```python
from build123d import *

# Parameters (mm, degrees)
MODEL_R             = 1.45
MODEL_RX            = 8.4
MODEL_RY            = 8
MODEL_W             = 3.6
MODEL_H             = 6.1
BOSS_EXTRUDE1_DEPTH = 5.85
FILLET1_R           = 0.3
FILLET2_R           = 1


with BuildPart() as part:
    # Model → Boss-Extrude1 (new body)
    with BuildSketch(Plane.XY):
        with BuildLine():
            Line((540.7427075, 594.649674665), (549.596103149, 594.649674665))
            Line((549.596103149, 594.649674665), (549.596103149, 592.109674665))
            Line((549.596103149, 592.109674665), (559.756103149, 592.109674665))
            Line((559.756103149, 592.109674665), (559.756103149, 594.649674665))
            Line((559.756103149, 594.649674665), (568.609498798, 594.649674665))
            ThreePointArc((568.609498798, 594.649674665), (575.419225536, 591.943953999), (578.10077955, 585.124674665))
            add(Edge.make_bspline(
                [(578.10077955, 585.124674665), (577.425296665, 565.444526899), (567.160030567, 565.124674665)],
                knots=[0, 0, 0, 1, 1, 1], degree=2))
            Line((567.160030567, 565.124674665), (542.192175731, 565.124674665))
            add(Edge.make_bspline(
                [(531.251426748, 585.124674665), (531.926909632, 565.444526899), (542.192175731, 565.124674665)],
                knots=[0, 0, 0, 1, 1, 1], degree=2))
            ThreePointArc((531.251426748, 585.124674665), (533.932980762, 591.943953999), (540.7427075, 594.649674665))
        make_face()
        with Locations((545.226103149, 571.324674665)):
            Circle(MODEL_R, mode=Mode.SUBTRACT)
        with Locations((564.126103149, 571.324674665)):
            Circle(MODEL_R, mode=Mode.SUBTRACT)
        with Locations(Location((541.476103149, 584.734674665), (0, 0, 180))):
            Ellipse(MODEL_RX, MODEL_RY, mode=Mode.SUBTRACT)
        with Locations(Location((567.876103149, 584.734674665), (0, 0, -180))):
            Ellipse(MODEL_RX, MODEL_RY, mode=Mode.SUBTRACT)
        with BuildLine():
            Line((549.856103149, 574.334674665), (554.676103149, 574.334674665))
            Line((554.676103149, 574.334674665), (559.496103149, 574.334674665))
            ThreePointArc((559.496103149, 574.334674665), (559.97693576, 574.533842054), (560.176103149, 575.014674665))
            Line((560.176103149, 575.014674665), (560.176103149, 578.654674665))
            ThreePointArc((560.176103149, 578.654674665), (559.97693576, 579.135507276), (559.496103149, 579.334674665))
            Line((559.496103149, 579.334674665), (554.676103149, 579.334674665))
            Line((554.676103149, 579.334674665), (549.856103149, 579.334674665))
            ThreePointArc((549.856103149, 579.334674665), (549.375270538, 579.135507276), (549.176103149, 578.654674665))
            Line((549.176103149, 578.654674665), (549.176103149, 575.014674665))
            ThreePointArc((549.176103149, 575.014674665), (549.375270538, 574.533842054), (549.856103149, 574.334674665))
        make_face(mode=Mode.SUBTRACT)
        with Locations((569.376103149, 571.324674665)):
            Rectangle(MODEL_W, MODEL_H, mode=Mode.SUBTRACT)
        with Locations((539.976103149, 571.324674665)):
            Rectangle(MODEL_W, MODEL_H, mode=Mode.SUBTRACT)
    extrude(amount=BOSS_EXTRUDE1_DEPTH)

    # Fillet1
    fillet1_edges = [part.edges().sort_by_distance(p)[0] for p in [
        (549.596103149, 592.109674665, 2.925),
        (559.756103149, 592.109674665, 2.925),
    ]]
    fillet(fillet1_edges, radius=FILLET1_R)

    # Fillet2
    fillet2_edges = [part.edges().sort_by_distance(p)[0] for p in [
        (549.596103149, 594.649674665, 2.925),
        (559.756103149, 594.649674665, 2.925),
    ]]
    fillet(fillet2_edges, radius=FILLET2_R)


solid = part.part
```
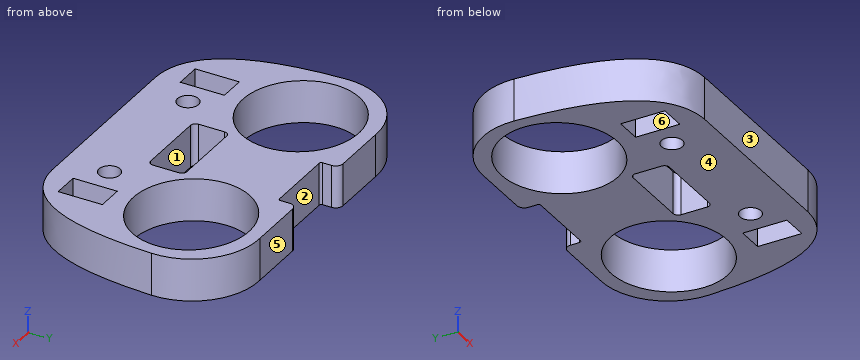
The listing builds one solid part. Answer for the finished solid, in the listing's coordinates (mm). Face numbers are marked on the shaded views. A direction names the side the tool comes from. Give positions to 0.01 mm unless a question says otherwise; leave off trailing zeros. Order: outer loops, then holes, each group sorted by start corner. A loop starts at its lowest first (then second) coordinate and runs counter-clockwise, first axis right, second up. Notation, with made-up numbers: (9.5, -32.75) -> (64.5, -32.75) arc R14 ccw to (64.5, -21.75) -> close; hole circle Ø11 at (-18.5, 16). An arc over 180 degrees is marked (long way). Answer as CSV lines item,"result". Start each with the question number.
Q1. A cutting plane is placed at A-A (x = 553). Determine the outline of the cut face in (y, z).
Q2. Find the intervals of material crossed by L1, parallel to X at y = 568.5, z = 1.1; L2, parallel to Y at x = 555.5, z = 3.65; L3, parallel to X at y = 572, z = 5.25, in increasing order.
Q3. A cutting plane is placed at B-B (y = 583.5). Count the separate pieces of the cut face and the enclosed holes in it, then the cut area to 3 significant figures.
Q4. Given pin 1 (1.1 mm diameter, centred on x = 540, z = 4, fed in from -Y); pin 2 (1.5 mm diameter, centred on x = 557, z = 0.5, fed in from +Y); pin 3 (1.4 mm diameter, centred on y = 593, z = 3, fed in from +X), each flat-ended and moving along its own axis, determine where each tip first touches the part or whether it passes through.
Q5. Determine the mould class of the marked faces 1, 2, 3 and 4 for opening direction Y: pulls with the +Y half, pulls with the -Y half, needs draft (parallel to the pull), parting line crosses it, or undercut.
Q6. Which of the six approach directions +Z, -Z, +X, -X, +Y, -Y give full straight-line access (tool end or side, diameter ignored) to the marked faces 5 and 6?
Results found:
1,outline,"(565.12, 0) -> (574.33, 0) -> (574.33, 5.85) -> (565.12, 5.85) -> close; (579.33, 0) -> (592.11, 0) -> (592.11, 5.85) -> (579.33, 5.85) -> close"
2,L1,"535.5 to 538.18, 541.78 to 567.58, 571.18 to 573.86"
2,L2,"565.12 to 574.33, 579.33 to 592.11"
2,L3,"533.51 to 538.18, 541.78 to 543.94, 546.51 to 562.84, 565.41 to 567.58, 571.18 to 575.84"
3,separate pieces,"3"
3,enclosed holes,"0"
3,area,"79.0 mm2"
4,pin 1,"y = 565.31"
4,pin 2,"y = 592.11"
4,pin 3,"x = 575.04"
5,face 1,"undercut"
5,face 2,"pulls with the +Y half"
5,face 3,"pulls with the -Y half"
5,face 4,"needs draft"
6,face 5,"+Z, -Z, +X, -X, +Y"
6,face 6,"+Z, -Z"
